Could you check a few things on this model? Use its own coordinates, in mm. Coordinates: 2 decimals unless noted, no trailing zeros. Loops run counter-clockwise (first coordinate to the right, second up) from the corner with the lowest first, then second, coordinate; pieces in that order, holes last. Notation, with made-up numbers: M 47.5,35.5 L 96.5,35.5 A18 ccw 96.5,56.5 Z; hole C -36.75,79 d5. An arc over 180 degrees is marked long. Use one line per item in the form item = value. Start each with the question number.
```python
from build123d import *

# Parameters (mm, degrees)
ESBO_O1_R                = 2.1
RESSALTO_EXTRUS_O1_DEPTH = 70


with BuildPart() as part:
    # Esboço1 → Ressalto-extrusão1 (new body)
    with BuildSketch(Plane.XY):
        with BuildLine():
            Line((3.9, -0.21), (3.69, 0))
            Line((3.69, 0), (3.9, 0.21))
            Line((3.9, 0.21), (3.9, 2.839339828))
            Line((3.9, 2.839339828), (6.560660172, 5.5))
            Line((6.560660172, 5.5), (8.2, 5.5))
            Line((8.2, 5.5), (8.2, 3.125))
            Line((8.2, 3.125), (8.545, 3.125))
            Line((8.545, 3.125), (10, 4.58))
            Line((10, 4.58), (10, 9.5))
            ThreePointArc((10, 9.5), (9.853553391, 9.853553391), (9.5, 10))
            Line((9.5, 10), (4.58, 10))
            Line((4.58, 10), (3.125, 8.545))
            Line((3.125, 8.545), (3.125, 8.2))
            Line((3.125, 8.2), (5.5, 8.2))
            Line((5.5, 8.2), (5.5, 6.560660172))
            Line((5.5, 6.560660172), (2.839339828, 3.9))
            Line((2.839339828, 3.9), (0.21, 3.9))
            Line((0.21, 3.9), (0, 3.69))
            Line((0, 3.69), (-0.21, 3.9))
            Line((-0.21, 3.9), (-2.839339828, 3.9))
            Line((-2.839339828, 3.9), (-5.5, 6.560660172))
            Line((-5.5, 6.560660172), (-5.5, 8.2))
            Line((-5.5, 8.2), (-3.125, 8.2))
            Line((-3.125, 8.2), (-3.125, 8.545))
            Line((-3.125, 8.545), (-4.58, 10))
            Line((-4.58, 10), (-9.5, 10))
            ThreePointArc((-9.5, 10), (-9.853553391, 9.853553391), (-10, 9.5))
            Line((-10, 9.5), (-10, 4.58))
            Line((-10, 4.58), (-8.545, 3.125))
            Line((-8.545, 3.125), (-8.2, 3.125))
            Line((-8.2, 3.125), (-8.2, 5.5))
            Line((-8.2, 5.5), (-6.560660172, 5.5))
            Line((-6.560660172, 5.5), (-3.9, 2.839339828))
            Line((-3.9, 2.839339828), (-3.9, 0.21))
            Line((-3.9, 0.21), (-3.69, 0))
            Line((-3.69, 0), (-3.9, -0.21))
            Line((-3.9, -0.21), (-3.9, -2.839339828))
            Line((-3.9, -2.839339828), (-6.560660172, -5.5))
            Line((-6.560660172, -5.5), (-8.2, -5.5))
            Line((-8.2, -5.5), (-8.2, -3.125))
            Line((-8.2, -3.125), (-8.545, -3.125))
            Line((-8.545, -3.125), (-10, -4.58))
            Line((-10, -4.58), (-10, -9.5))
            ThreePointArc((-10, -9.5), (-9.853553391, -9.853553391), (-9.5, -10))
            Line((-9.5, -10), (-4.58, -10))
            Line((-4.58, -10), (-3.125, -8.545))
            Line((-3.125, -8.545), (-3.125, -8.2))
            Line((-3.125, -8.2), (-5.5, -8.2))
            Line((-5.5, -8.2), (-5.5, -6.560660172))
            Line((-5.5, -6.560660172), (-2.839339828, -3.9))
            Line((-2.839339828, -3.9), (-0.21, -3.9))
            Line((-0.21, -3.9), (0, -3.69))
            Line((0, -3.69), (0.21, -3.9))
            Line((0.21, -3.9), (2.839339828, -3.9))
            Line((2.839339828, -3.9), (5.5, -6.560660172))
            Line((5.5, -6.560660172), (5.5, -8.2))
            Line((5.5, -8.2), (3.125, -8.2))
            Line((3.125, -8.2), (3.125, -8.545))
            Line((3.125, -8.545), (4.58, -10))
            Line((4.58, -10), (9.5, -10))
            ThreePointArc((9.5, -10), (9.853553391, -9.853553391), (10, -9.5))
            Line((10, -9.5), (10, -4.58))
            Line((10, -4.58), (8.545, -3.125))
            Line((8.545, -3.125), (8.2, -3.125))
            Line((8.2, -3.125), (8.2, -5.5))
            Line((8.2, -5.5), (6.560660172, -5.5))
            Line((6.560660172, -5.5), (3.9, -2.839339828))
            Line((3.9, -2.839339828), (3.9, -0.21))
        make_face()
        Circle(ESBO_O1_R, mode=Mode.SUBTRACT)
    extrude(amount=RESSALTO_EXTRUS_O1_DEPTH)


solid = part.part
```
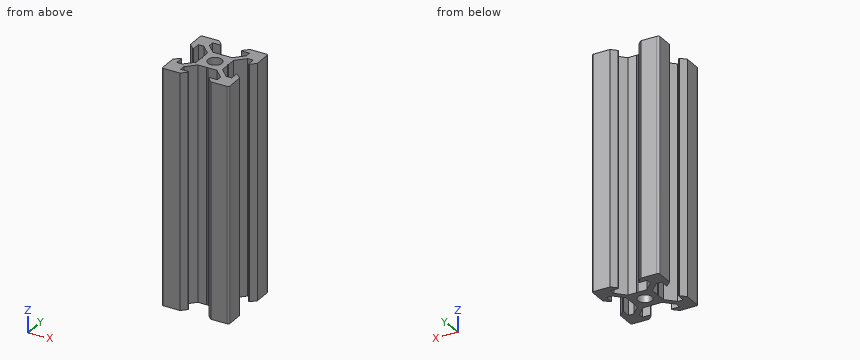
Item 1: Please list where these lines run through material, in increasing order: line 1 along X through (y, z) = (7.75, 15); line 2 along Y through (x, z) = (4.25, 46).
Item 2: I'm going to push flat-ended pins straight in: P1, Ø0.8, axis at x = -1, z = 46.5, coming from the +Y side; P2, Ø2.5, axis at x = 4, z = 28.5, coming from the +Y side; P3, Ø3, axis at x = 1, z = 21.5, coming from the -Y side; P4, Ø2, axis at y = -2.5, z = 14, coming from the -X side. Where does each tip first touch, or does it pass through?
Item 3: I want a section at A-A (y = -1.25). Write out the boundary of the cut face in (x, z), plus the area to 3 significant figures.
Worked answers:
q1.line_1 = -10 to -5.5, 5.5 to 10
q1.line_2 = -9.67 to -8.2, -5.31 to -3.19, 3.19 to 5.31, 8.2 to 9.67
q2.P1 = 3.9
q2.P2 = 10
q2.P3 = -3.9
q2.P4 = -8.92
q3.outline = M -3.9,0 L -1.69,0 L -1.69,70 L -3.9,70 Z; M 1.69,0 L 3.9,0 L 3.9,70 L 1.69,70 Z
q3.area = 310 mm²
